from build123d import *

# Parameters (mm, degrees)
SKETCH_1_W      = 46
SKETCH_1_H      = 24
EXTRUDE_1_DEPTH = 9
SKETCH_4_R      = 1.5
EXTRUDE_2_DEPTH = 9
FILLET_1_R      = 2


with BuildPart() as part:
    # Эскиз1 → Бобышка-Вытянуть1 (new body)
    with BuildSketch(Plane.XY):
        Rectangle(SKETCH_1_W, SKETCH_1_H)
    extrude(amount=EXTRUDE_1_DEPTH)

    # Эскиз2 → По сечениям1 section 0
    with BuildSketch(Plane.XY.offset(9)):
        with BuildLine():
            Line((-23, 12), (-6, 12))
            Line((-6, 12), (-6, -12))
            Line((-6, -12), (-23, -12))
            Line((-23, -12), (-23, 12))
        make_face()
    # Эскиз3 → По сечениям1 section 1
    with BuildSketch(Plane.XY.offset(14)):
        with BuildLine():
            Line((-23, 12), (-10, 12))
            Line((-10, 12), (-10, -12))
            Line((-10, -12), (-23, -12))
            Line((-23, -12), (-23, 12))
        make_face()
    loft()

    # Эскиз4 → Бобышка-Вытянуть2 (add)
    with BuildSketch(Plane(origin=(23, 0, 0), x_dir=(0, 0, -1), z_dir=(1, 0, 0))):
        with Locations(Location((-2.128573829, 0, 0), (0, 0, 270))):
            Circle(SKETCH_4_R)
    extrude(amount=EXTRUDE_2_DEPTH)

    # Скругление1
    fillet_1_edges = [part.edges().sort_by_distance(p)[0] for p in [
        (-6, 0, 9),
        (23, -12, 4.5),
        (23, 12, 4.5),
    ]]
    fillet(fillet_1_edges, radius=FILLET_1_R)


solid = part.part
Build history of the part. All positions in model axes, mm. A direction names the side the tool comes from. Coordinates: 2 decimals unless noted, no trailing zeros. Order: outer loops, then holes, each group sorted by start corner. A loop starts at its lowest first (then second) coordinate and runs counter-clockwise, first axis right, second up. Notation, with made-up numbers: M 1.25,-6.75 L 49.25,-6.75 A20 ccw 49.25,-1.75 Z; hole C 38.25,-4 d4. An arc over 180 degrees is marked long. One line per question, with ' | ' between items. Start each with the question number.
Q1. Probe L1, parallel to X at y = 7.75, z = 5.25; L2, parallel to Z at x = 10, y = -4.25; L3, parallel to X at y = -10.25, z = 10.5. List the from-to ranges inside material, lowest first. Write a range as from..to.
Q2. Saw through at D-D (y = 0). List the corners of the cut face in (x, z), then the cut area to 3 significant figures.
Q3. 3-axis set-ups, long thin cutter, end or side, ignore diameter. For faces 1 (the face through (27.44, 0.2, 0.64)), 2 (the face through (0, 0, 0)), 3 (the face through (9, 0, 9)): which of +Z, -Z, +X, -X, +Y, -Y reach the whole face in a straight line?
Q4. Saw through at B-B (z = 5). List the corners of the cut face in (x, y).
Q5. Flat gauge pin, fed straight in: pin 1 Ø7 at (y, z) = (-4, 6.5) entering from +X. Where does the tip first touch, or does it go through?
Q6. Saw through at C-C (x = 15). List the corners of the cut face in (y, z), then the cut area to 3 significant figures.
Q7. Saw through at A-A (y = 3.5). List the corners of the cut face in (x, z).
Check values:
1) L1: x = -23..23 | L2: z = 0..9 | L3: x = -23..-7.2
2) outline: M -23,0 L 23,0 L 23,0.63 L 32,0.63 L 32,3.63 L 23,3.63 L 23,9 L -5.04,9 A2 cw -6.6,9.75 L -10,14 L -23,14 Z | area: 516 mm2
3) face 1: +X | face 2: -Z, +X, -X, +Y, -Y | face 3: +Z, +X, +Y, -Y
4) outline: M -23,-12 L 21,-12 A2 ccw 23,-10 L 23,10 A2 ccw 21,12 L -23,12 Z
5) pin 1: stops at x = 23
6) outline: M -12,0 L 12,0 L 12,9 L -12,9 Z | area: 216 mm2
7) outline: M -23,0 L 23,0 L 23,9 L -5.04,9 A2 cw -6.6,9.75 L -10,14 L -23,14 Z
